Can you work these out from the model? Positions are in its coordinate system, mm. A direction names the side the tool comes from. Give positions to 0.01 mm unless a question says otherwise; leave off trailing zeros. Order: outer loops, then holes, each group sorted by start corner. A loop starts at its lowest first (then second) coordinate and runs counter-clockwise, first axis right, second up. Notation, with made-up numbers: (-30, 30.5) -> (17, 30.5) arc R27 ccw to (17, 52.5) -> close; hole circle Ø5 at (19, 88.5). An arc over 180 degrees is marked (long way). Answer as CSV lines item,"result".
```python
from build123d import *

# Parameters (mm, degrees)
EXTRUDE_1_DEPTH      = 10
EXTRUDE_1_DEPTH_BACK = 10.26
SKETCH_4_R           = 17.9
EXTRUDE_3_DEPTH      = 60
EXTRUDE_7_DEPTH      = 16.5
EXTRUDE_7_DEPTH_BACK = 16.5
SKETCH_15_R          = 6
SKETCH_17_R          = 3.25
CUT_EXTRUDE_3_DEPTH  = 13
CUT_EXTRUDE_4_DEPTH  = 1.95
FILLET_1_R           = 3
HOLE_WIZARD_M2_5_1_D = 2.9
CHAMFER_1_SIZE       = 1


with BuildPart() as part:
    # 스케치1 → 보스-돌출1 (new, two sides: drawn at the far end of the back side and taken through both)
    with BuildSketch(Plane(origin=(0, 0, 0), x_dir=(0, 0, -1), z_dir=(1, 0, 0)).offset(-EXTRUDE_1_DEPTH_BACK)):
        with BuildLine():
            Line((20, -24), (20, 0))
            ThreePointArc((20, 0), (0, 20), (-20, 0))
            Line((-20, 0), (-20, -24))
            Line((-20, -24), (20, -24))
        make_face()
    extrude(amount=EXTRUDE_1_DEPTH + EXTRUDE_1_DEPTH_BACK)

    # 스케치4 → 보스-돌출3 (add)
    with BuildSketch(Plane.ZY.offset(10.26)):
        Circle(SKETCH_4_R)
    extrude(amount=EXTRUDE_3_DEPTH)

    # 스케치15 → 보스-돌출7 (add, two sides: drawn at the far end of the back side and taken through both)
    with BuildSketch(Plane.XY.offset(-EXTRUDE_7_DEPTH_BACK)):
        with BuildLine():
            Line((-6, -24), (-6, -30))
            ThreePointArc((-6, -30), (-4.242640687, -25.757359313), (0, -24))
            Line((0, -24), (-6, -24))
        make_face()
        with Locations((0, -30)):
            Circle(SKETCH_15_R)
        with BuildLine():
            ThreePointArc((0, -24), (4.242640687, -25.757359313), (6, -30))
            Line((6, -30), (6, -24))
            Line((6, -24), (0, -24))
        make_face()
    extrude(amount=EXTRUDE_7_DEPTH + EXTRUDE_7_DEPTH_BACK)

    # 스케치17 → 컷-돌출3 (cut)
    with BuildSketch(Plane(origin=(0, 0, -16.5), x_dir=(-1, 0, 0), z_dir=(0, 0, -1))):
        with Locations((0, -30)):
            Circle(SKETCH_17_R)
    cut_extrude_3 = extrude(amount=-CUT_EXTRUDE_3_DEPTH, mode=Mode.SUBTRACT)

    # 대칭 복사7: 컷-돌출3 across plane
    add(cut_extrude_3.mirror(Plane.XY), mode=Mode.SUBTRACT)

    # 스케치18 → 컷-돌출4 (cut, symmetric)
    with BuildSketch(Plane(origin=(0, 0, -10.5), x_dir=(-1, 0, 0), z_dir=(0, 0, -1))):
        Polygon((-4.2, -36), (4.2, -36), (4.2, -32.424871131), (0, -34.849742261), (-4.2, -32.424871131), align=None)
        Polygon((-4.2, -27.575128869), (-4.2, -32.424871131), (0, -34.849742261), (4.2, -32.424871131), (4.2, -27.575128869), (0, -25.150257739), align=None)
    cut_extrude_4 = extrude(amount=CUT_EXTRUDE_4_DEPTH, both=True, mode=Mode.SUBTRACT)

    # 대칭 복사8: 컷-돌출4 across plane
    add(cut_extrude_4.mirror(Plane.XY), mode=Mode.SUBTRACT)

    # 필렛1
    fillet_1_edges = [part.edges().sort_by_distance(p)[0] for p in [
        (-6, -24, 0),
        (6, -24, 0),
    ]]
    fillet(fillet_1_edges, radius=FILLET_1_R)

    # M2.5 여유 구멍1 (through all)
    with Locations(Plane(origin=(0, 17.9, 0), x_dir=(1, 0, 0), z_dir=(0, 1, 0))):
        with Locations((-35.26, 0)):
            Hole(HOLE_WIZARD_M2_5_1_D / 2)

    # 모따기1
    chamfer_1_edges = [part.edges().sort_by_distance(p)[0] for p in [
        (-70.26, 0, -17.9),
    ]]
    chamfer(chamfer_1_edges, length=CHAMFER_1_SIZE)


solid = part.part
```
Item 1: Imagine slicing it at C-C, the plane x = -35.26. Please give me the cut outline in (y, z).
Numbers:
outline,"(-17.84, -1.45) arc R17.9 ccw to (17.84, -1.45) -> close; (-17.84, 1.45) -> (17.84, 1.45) arc R17.9 ccw to start"
Item 2: For faces 5 (the flat face through (-4.2, -31, 11)), 6 (the flat face through (0, -30, -3.5)), 7 (the cylindrical face through (0.705, -33.173, 6.06)), 8 (the flat face through (6, -29, 0)), which set-ups out of +Z, -Z, +X, -X, +Y, -Y let a thin tool reach every point of the face, with its end or its side?
Numbers:
face 5,"-Y"
face 6,"-Z"
face 7,"+Z"
face 8,"+Z, -Z, +X, -Y"
Item 3: For pin 1 (8.5 mm diameter, centred on x = 0, y = -30, fed in from -Z); pin 2 (4 mm diameter, centred on x = -48.5, y = 1.5, fed in from -Z); pin 3 (4.5 mm diameter, centred on y = -31.5, z = 11, fed in from -X), each with a flat end and sliding along its axis, tell me the tip position at first contact or that it passes through.
Numbers:
pin 1,"stops at z = -16.5"
pin 2,"stops at z = -17.9"
pin 3,"stops at x = -6"
Item 4: We'd pull the mould along X, two halves only. Please class faces 1 (the flat face through (2.071, -26.346, 10.527)), 2 (the flat face through (-10.26, -18, 2)), 3 (the flat face through (0, -12, -20)), 4 (the flat face through (-2, -33, -8.55)): released by +X, released by -X, zero draft, split by the parting line, or undercut.
Numbers:
face 1,"undercut"
face 2,"released by -X"
face 3,"zero draft"
face 4,"undercut"
Item 5: Imagine slicing it at B-B, the plane x = -16. Please give me the cut outline in (y, z).
Numbers:
outline,"circle Ø35.8 at (0, 0)"
Item 6: Please list where these lines run through material, in increasing order: line 1 along X through (y, z) = (-30, 7.3); line 2 along X through (y, z) = (14, -11.5); line 3 along Y through (x, z) = (0, -15).
Numbers:
line 1,"x = -6 to -3.25, 3.25 to 6"
line 2,"x = -10.26 to 10"
line 3,"y = -36 to -33.25, -26.75 to 13.23"
Item 7: Imagine slicing it at A-A, the plane y = -28.5. Please give me the cut outline in (x, z).
Numbers:
outline,"(-6, -16.5) -> (-2.88, -16.5) -> (-2.88, -12.45) -> (-4.2, -12.45) -> (-4.2, -8.55) -> (-2.88, -8.55) -> (-2.88, -3.5) -> (2.88, -3.5) -> (2.88, -8.55) -> (4.2, -8.55) -> (4.2, -12.45) -> (2.88, -12.45) -> (2.88, -16.5) -> (6, -16.5) -> (6, 16.5) -> (2.88, 16.5) -> (2.88, 12.45) -> (4.2, 12.45) -> (4.2, 8.55) -> (2.88, 8.55) -> (2.88, 3.5) -> (-2.88, 3.5) -> (-2.88, 8.55) -> (-4.2, 8.55) -> (-4.2, 12.45) -> (-2.88, 12.45) -> (-2.88, 16.5) -> (-6, 16.5) -> close"
